from build123d import *

# Parameters (mm, degrees)
BOSS_EXTRU_1_DEPTH      = 2
BOSS_EXTRU_1_DEPTH_BACK = 1
ESQUISSE1_W             = 32
ESQUISSE1_H             = 3
D_GAGEMENT_M1_61_D      = 1.6


with BuildPart() as part:
    # Esquisse1 → Boss.-Extru.1 (new, two sides: drawn at the far end of the back side and taken through both)
    with BuildSketch(Plane(origin=(0, 0, 0), x_dir=(1, 0, 0), z_dir=(0, 1, 0)).offset(-BOSS_EXTRU_1_DEPTH_BACK)):
        with Locations((16, 1.5)):
            Rectangle(ESQUISSE1_W, ESQUISSE1_H)
    extrude(amount=BOSS_EXTRU_1_DEPTH + BOSS_EXTRU_1_DEPTH_BACK)

    # Dégagement M1.61 (through all)
    with Locations(Plane(origin=(16, 0.5, 0), x_dir=(1, 0, 0), z_dir=(0, 0, 1))):
        with Locations((0, 0)):
            Hole(D_GAGEMENT_M1_61_D / 2)


solid = part.part
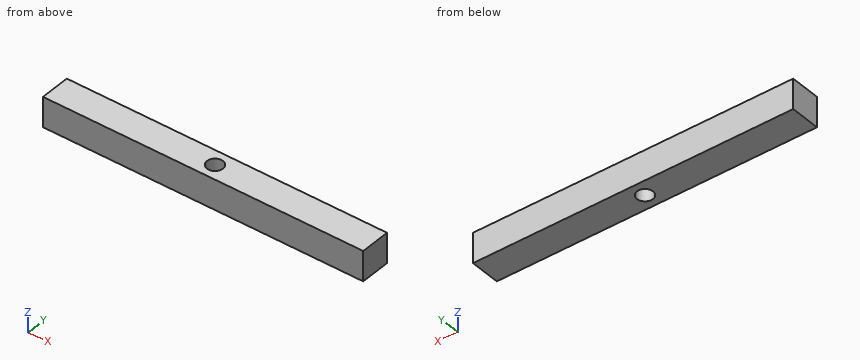
Geometry: final body of the model. Coordinates: model frame, mm. Round coordinates to 2 decimals unless told otherwise and drop trailing zeros. Loops run counter-clockwise (first coordinate to the right, second up) from the corner with the lowest first, then second, coordinate; pieces in that order, holes last. Notation, with made-up numbers: M 47,20 L 97,20 A27 cw 97,46 Z; hole C 9.25,44.25 d8. An arc over 180 degrees is marked long. One line per question, with ' | ' between items.
(1) Contact query for a flat-ended pin moving along its axis: P1, Ø1, axis at x = 16, y = 0.5, coming from the +Z side. Output: stop coordinate, or through.
Check result:
P1: passes through
(2) Cut plane C-C on z = -1.3. Return the cut outline in (x, y).
Check result:
outline: M 0,-1 L 32,-1 L 32,2 L 0,2 Z; hole C 16,0.5 d1.6
(3) Cut plane B-B on x = 16. Return the cut outline in (y, z).
Check result:
outline: M -1,-3 L -0.3,-3 L -0.3,0 L -1,0 Z; M 1.3,-3 L 2,-3 L 2,0 L 1.3,0 Z
(4) Cut plane A-A on y = 0.5. Return the cut outline in (x, z).
Check result:
outline: M 0,-3 L 15.2,-3 L 15.2,0 L 0,0 Z; M 16.8,-3 L 32,-3 L 32,0 L 16.8,0 Z
(5) Material intervals for line 1 along Y through (x, z) = (16, -0.7); line 2 along X through (y, z) = (0.35, -2.3); line 3 along X through (y, z) = (-0.05, -0.65), sorted ascending. Write a range as from..to.
Check result:
line 1: y = -1..-0.3, 1.3..2 | line 2: x = 0..15.21, 16.79..32 | line 3: x = 0..15.42, 16.58..32
